Input: dimensioned drawing with shaded views. Units: mm. Origin: part minimum x, y, z. A direction names the side the tool comes from. Coordinates: 2 decimals unless noted, no trailing zeros. Loops run counter-clockwise (first coordinate to the right, second up) from the corner with the lowest first, then second, coordinate; pieces in that order, holes last. Notation, with made-up numbers: (33, -36) -> (78, -36) arc R30 cw to (78, -5) -> close; hole circle Ø5 at (-6.5, -15.75). An arc over 180 degrees is marked (long way). Answer as CSV lines item,"result".
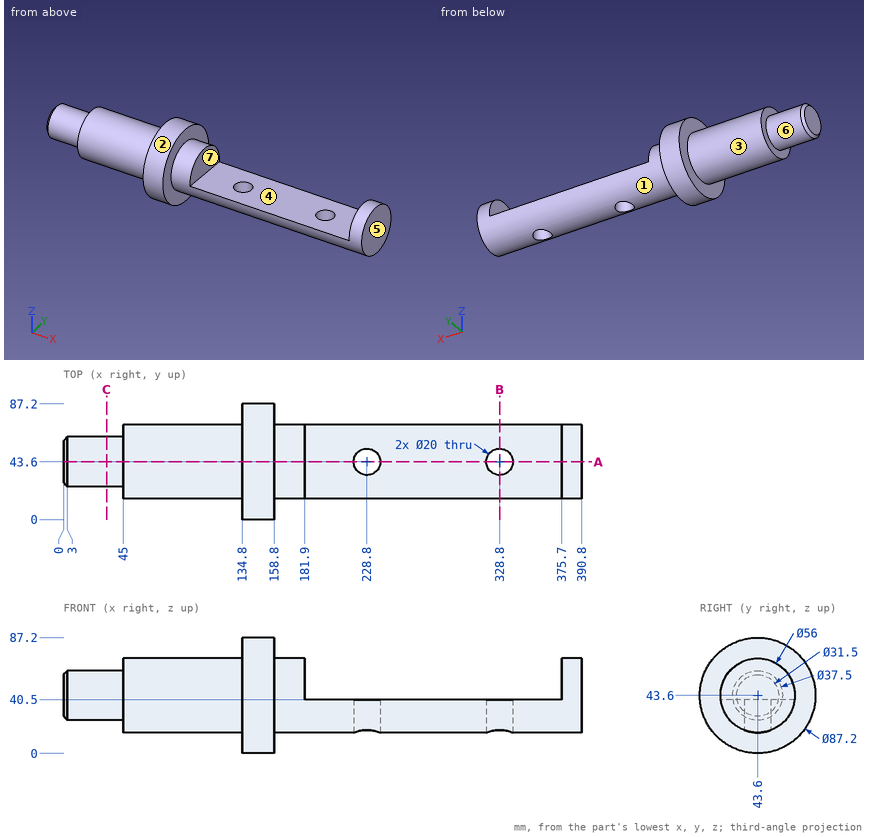
(1) Draft query along X for the marked faces 4, 5, 6 and 7. Return one class per face: released by +X, released by -X, zero draft, split by the parting line, or undercut.
Computed values:
face 4,"undercut"
face 5,"released by +X"
face 6,"zero draft"
face 7,"undercut"
(2) Cut plane C-C (x = 32.5). Return the cut outline in (y, z), then the cut area to 3 significant figures.
Computed values:
outline,"circle Ø37.5 at (43.6, 43.6)"
area,"1,100 mm^2"
(3) Pin query (flat end, axial travel): pin 1 Ø2 at (x, z) = (144.5, 25.5) entering from +Y; pin 2 Ø18 at (x, y) = (228.8, 43.6) entering from +Z; pin 3 Ø1 at (y, z) = (9.5, 25) entering from +X; pin 4 Ø2 at (x, y) = (68, 25) entering from +Z. Return the tip coordinate at first contact, or that it passes through.
Computed values:
pin 1,"y = 83.71"
pin 2,"through"
pin 3,"x = 158.8"
pin 4,"z = 65.38"
(4) Access query for the marked faces 1, 2 and 3. Directions: +Z, -Z, +X, -X, +Y, -Y. A direction counts if a zero-diameter tool reaches every point of the face in a straight line with its end or side. Return the directions, or none.
Computed values:
face 1,"+X"
face 2,"+X, -X"
face 3,"-X"
(5) Cut plane B-B (x = 328.8). Return the cut outline in (y, z), then the cut area to 3 significant figures.
Computed values:
outline,"(15.77, 40.5) arc R28 ccw to (33.6, 17.45) -> (33.6, 40.5) -> close; (53.6, 17.45) arc R28 ccw to (71.43, 40.5) -> (53.6, 40.5) -> close"
area,"572 mm^2"
(6) Cut plane A-A (y = 43.6). State how many separate pieces and enclosed holes the cut face has, then the cut area to 3 significant figures.
Computed values:
separate pieces,"3"
enclosed holes,"0"
area,"14,800 mm^2"
(7) Material intervals for L1, parallel to X at y = 43.6, z = 31.5; L2, parallel to X at y = 43, z = 27; L3, parallel to X at y = 78.5, z = 40.5, sorted ascending. Write a range as [from, to].
Computed values:
L1,"[0, 218.8], [238.8, 318.8], [338.8, 390.8]"
L2,"[0.86, 218.82], [238.78, 318.82], [338.78, 390.8]"
L3,"[134.8, 158.8]"
